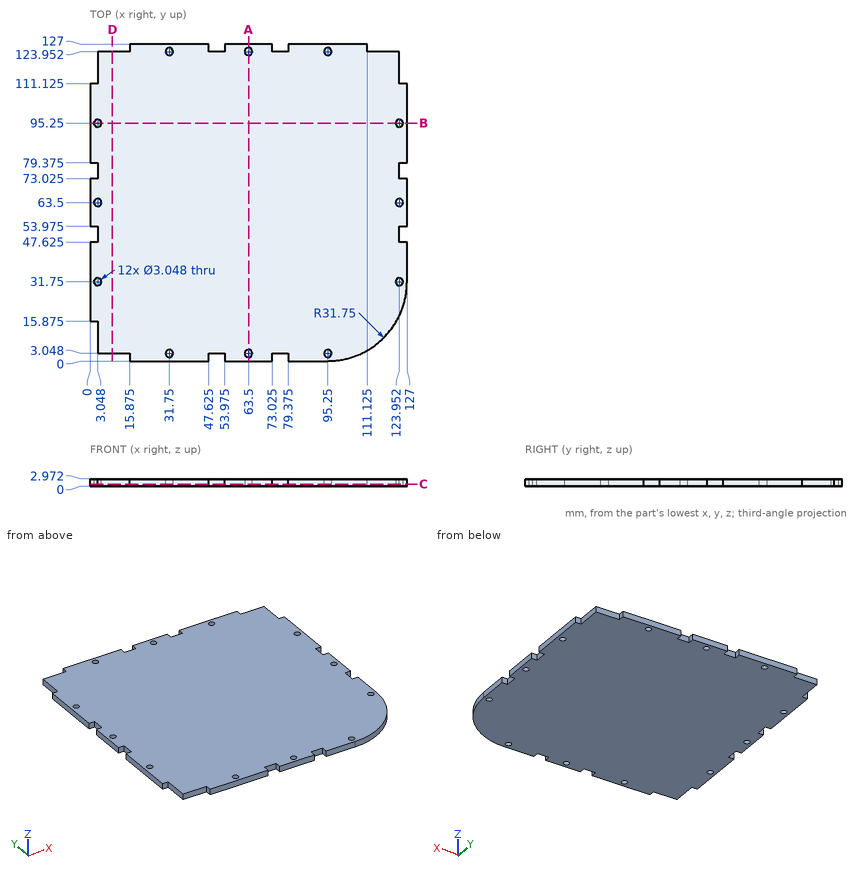
Input: dimensioned drawing with shaded views. Units: mm. Origin: part minimum x, y, z. Coordinates: 2 decimals unless noted, no trailing zeros. Write each loop counter-clockwise with the first axis right and the second up, starting at its lowest first coordinate (ties: lowest second). Pieces come first, ordered by that corner, then holes. Notation, with made-up numbers: M -36.75,12 L -1.75,12 A9 ccw -1.75,23 Z; hole C 85,35 d2. An arc over 180 degrees is marked long. Answer as CSV lines item,"result". Start each with the question number.
Q1. Cut plane C-C on z = 0.95. Count the separate pieces of the cut face and the enclosed holes in it, then the cut area to 3 significant figures.
Q2. Cut plane A-A on x = 63.5. Return the cut outline in (y, z), then the cut area to 3 significant figures.
Q3. Pin query (flat end, axial travel): P1, Ø0.9, axis at x = 124.5, z = 2, coming from the -Y side (1 decimal); P2, Ø1.5, axis at y = 7.5, z = 1.5, coming from the -X side; P3, Ø0.9, axis at y = 1, z = 2, coming from the -X side (3 decimals). Return the tip coordinate at first contact, or that it passes through.
Q4. Cut plane D-D on x = 9. Return the cut outline in (y, z).
Q5. Line query: line 1 (Y direction, x = 31.75, z = 1.1); line 2 (Y direction, x = 6.5, z = 1.8). Output: solid intervals per line, ascending. Write a range as from..to.
Findings below:
1,separate pieces,"1"
1,enclosed holes,"12"
1,area,"15,400 mm2"
2,outline,"M 0,0 L 1.52,0 L 1.52,2.97 L 0,2.97 Z; M 4.57,0 L 122.43,0 L 122.43,2.97 L 4.57,2.97 Z; M 125.48,0 L 127,0 L 127,2.97 L 125.48,2.97 Z"
2,area,"359 mm2"
3,P1,"stops at y = 18.4"
3,P2,"stops at x = 3.05"
3,P3,"stops at x = 15.875"
4,outline,"M 3.05,0 L 123.95,0 L 123.95,2.97 L 3.05,2.97 Z"
5,line 1,"y = 0..1.52, 4.57..122.43, 125.48..127"
5,line 2,"y = 3.05..123.95"
